Can you work these out from the drawing? Everything is in mm from the part's minimum corner. Round coordinates to 2 decimals unless told otherwise and drop trailing zeros. Loops run counter-clockwise (first coordinate to the right, second up) from the corner with the lowest first, then second, coordinate; pieces in that order, holes last. Notation, with made-up numbers: (-17.75, 24) - (-9.75, 24) arc R17 cw to (-9.75, 53) - close; hole circle Ø10 at (-13, 74). An arc over 180 degrees is marked (long way). Put each result on its own line as item: value. Start each with the question number.
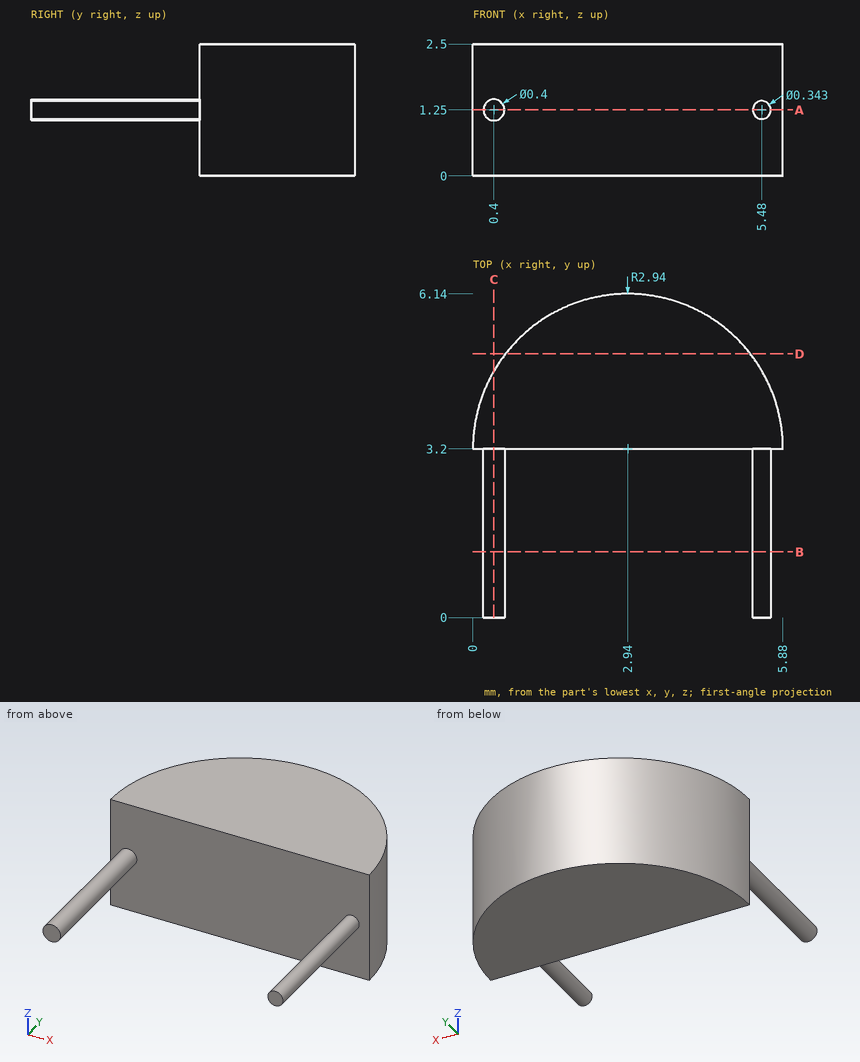
Item 1: Suppose I cut it at B-B, the plane y = 1.25. List the corners of the cut face in (x, z) for me.
Item 2: Suppose I cut it at C-C, the plane x = 0.4. List the corners of the cut face in (y, z) for me.
Item 3: Will this pin go through, and if not, where does the flat tip stop? P1, Ø0.8, axis at x = 2, z = 2, coming from the -Y side.
Item 4: I need wall thicknesses on line 1 (X direction, y = 2.25, z = 1.15); line 2 (Y direction, x = 3.9, z = 2.05); line 3 (X direction, y = 4.5, z = 1.85). Which ranges of each line are inside material? Lowest first, please. Write a range as from..to.
Item 5: Suppose I cut it at A-A, the plane z = 1.25. List the corners of the cut face in (x, y) for me.
Item 6: Suppose I cut it at D-D, the plane y = 5. List the corners of the cut face in (x, z) for me (1 decimal).
Numbers:
1. outline: circle Ø0.4 at (0.4, 1.25); circle Ø0.34 at (5.48, 1.25)
2. outline: (0, 1.05) - (3.2, 1.05) - (3.2, 0) - (4.68, 0) - (4.68, 2.5) - (3.2, 2.5) - (3.2, 1.45) - (0, 1.45) - close
3. P1: y = 3.2
4. line 1: 0.23..0.57, 5.34..5.62
4. line 2: 3.2..5.98
4. line 3: 0.3..5.58
5. outline: (0, 3.2) - (0.2, 3.2) - (0.2, 0) - (0.6, 0) - (0.6, 3.2) - (5.31, 3.2) - (5.31, 0) - (5.65, 0) - (5.65, 3.2) - (5.88, 3.2) arc R2.94 ccw to start
6. outline: (0.6, 0) - (5.3, 0) - (5.3, 2.5) - (0.6, 2.5) - close
